Could you check a few things on this model? Use its own coordinates, in mm. Give positions to 0.01 mm unless a question says otherwise; leave off trailing zeros. Order: outer loops, then holes, each group sorted by start corner. A loop starts at its lowest first (then second) coordinate and runs counter-clockwise, first axis right, second up.
(1) If I drill on probe 1 along Y at (x, z) = (7.5, 3); probe 2 along Y at (x, z) = (58.55, 1.75); probe 3 along Y at (x, z) = (99.5, 1.5), over which ranges is the centre line in solid material (lowest first)?
(2) Imagine slicing it at B-B, the plane x = 207.01. Write out the boundary of the cut face in (y, z) (3 decimals), then the cut area to 3 significant figures.
(3) Imagine slicing it at A-A, the plane y = 44.9. State how many separate pieces and enclosed holes the cut face has, then the cut area to 3 significant figures.
(4) Imagine slicing it at D-D, the plane x = 149. Write out the boundary of the cut face in (y, z), then the cut area to 3 significant figures.
(5) Imagine slicing it at C-C, the plane y = 34. Write out the boundary of the cut face in (x, z), then the cut area to 3 significant figures.
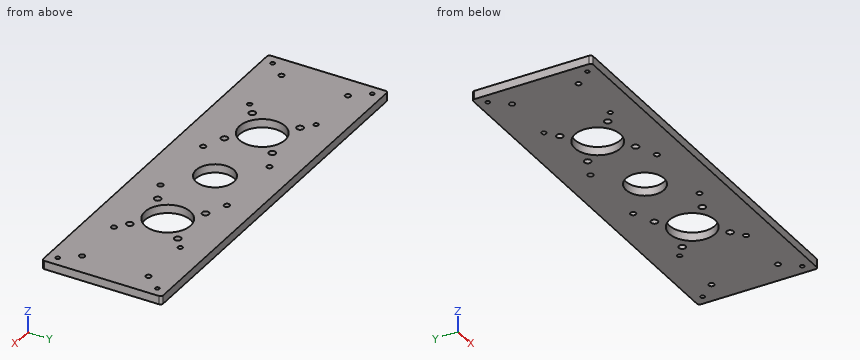
from build123d import *

# Parameters (mm, degrees)
SKETCH1_W           = 292.1
SKETCH1_H           = 89.8
SKETCH1_R           = 14.2875
SKETCH1_R_2         = 2.54
SKETCH1_R_3         = 17.145
BOSS_EXTRUDE1_DEPTH = 6.35
SKETCH2_R           = 2.05
CUT_EXTRUDE1_DEPTH  = 10
SKETCH3_R           = 1.55
SKETCH3_R_2         = 2.05
CUT_EXTRUDE2_DEPTH  = 10
FILLET1_R           = 2
SKETCH4_R           = 2.05
SKETCH4_R_2         = 1.778
CUT_EXTRUDE4_DEPTH  = 7.35


with BuildPart() as part:
    # Sketch1 → Boss-Extrude1 (new body)
    with BuildSketch(Plane.XY):
        with Locations((146.05, 44.9)):
            Rectangle(SKETCH1_W, SKETCH1_H)
        with Locations((146.05, 44.9)):
            Circle(SKETCH1_R, mode=Mode.SUBTRACT)
        with Locations((103.051585406, 62.859439014)):
            Circle(SKETCH1_R_2, mode=Mode.SUBTRACT)
        with Locations((103.049439014, 26.938414594)):
            Circle(SKETCH1_R_2, mode=Mode.SUBTRACT)
        with Locations((67.128414594, 26.940560986)):
            Circle(SKETCH1_R_2, mode=Mode.SUBTRACT)
        with Locations((67.130560986, 62.861585406)):
            Circle(SKETCH1_R_2, mode=Mode.SUBTRACT)
        with Locations((85.09, 44.9)):
            Circle(SKETCH1_R_3, mode=Mode.SUBTRACT)
        with Locations((189.050560986, 62.861585406)):
            Circle(SKETCH1_R_2, mode=Mode.SUBTRACT)
        with Locations((224.971585406, 62.859439014)):
            Circle(SKETCH1_R_2, mode=Mode.SUBTRACT)
        with Locations((224.969439014, 26.938414594)):
            Circle(SKETCH1_R_2, mode=Mode.SUBTRACT)
        with Locations((189.048414594, 26.940560986)):
            Circle(SKETCH1_R_2, mode=Mode.SUBTRACT)
        with Locations((207.01, 44.9)):
            Circle(SKETCH1_R_3, mode=Mode.SUBTRACT)
    extrude(amount=BOSS_EXTRUDE1_DEPTH)

    # Sketch2 → Cut-Extrude1 (cut)
    with BuildSketch(Plane.XY.offset(6.35)):
        with Locations((118.55, 20)):
            Circle(SKETCH2_R)
        with Locations((118.55, 69.8)):
            Circle(SKETCH2_R)
        with Locations((173.55, 20)):
            Circle(SKETCH2_R)
        with Locations((173.55, 69.8)):
            Circle(SKETCH2_R)
    extrude(amount=-CUT_EXTRUDE1_DEPTH, mode=Mode.SUBTRACT)

    # Sketch3 → Cut-Extrude2 (cut)
    with BuildSketch(Plane.XY.offset(6.35)):
        with Locations((284.6, 7.5)):
            Circle(SKETCH3_R)
        with Locations((7.5, 7.5)):
            Circle(SKETCH3_R)
        with Locations((7.5, 82.3)):
            Circle(SKETCH3_R)
        with Locations((284.6, 82.3)):
            Circle(SKETCH3_R)
        with Locations((274.6, 20)):
            Circle(SKETCH3_R_2)
        with Locations((17.5, 20)):
            Circle(SKETCH3_R_2)
        with Locations((17.5, 69.8)):
            Circle(SKETCH3_R_2)
        with Locations((274.6, 69.8)):
            Circle(SKETCH3_R_2)
    extrude(amount=-CUT_EXTRUDE2_DEPTH, mode=Mode.SUBTRACT)

    # Fillet1
    fillet1_edges = [part.edges().sort_by_distance(p)[0] for p in [
        (0, 89.8, 3.175),
        (292.1, 89.8, 3.175),
        (292.1, 0, 3.175),
        (0, 0, 3.175),
    ]]
    fillet(fillet1_edges, radius=FILLET1_R)

    # Sketch4 → Cut-Extrude4 (cut, through all)
    with BuildSketch(Plane.XY.offset(6.35)):
        with Locations((233.55, 20)):
            Circle(SKETCH4_R)
        with Locations((233.55, 69.8)):
            Circle(SKETCH4_R_2)
        with Locations((58.55, 69.8)):
            Circle(SKETCH4_R_2)
        with Locations((58.55, 20)):
            Circle(SKETCH4_R_2)
    extrude(amount=-CUT_EXTRUDE4_DEPTH, mode=Mode.SUBTRACT)


solid = part.part
Answer block:
1. probe 1: y = 0 to 5.95, 9.05 to 80.75, 83.85 to 89.8
1. probe 2: y = 0 to 18.22, 21.78 to 68.02, 71.58 to 89.8
1. probe 3: y = 0 to 35.61, 54.19 to 89.8
2. outline: (0, 0) - (27.755, 0) - (27.755, 6.35) - (0, 6.35) - close; (62.045, 0) - (89.8, 0) - (89.8, 6.35) - (62.045, 6.35) - close
2. area: 352 mm2
3. separate pieces: 4
3. enclosed holes: 0
3. area: 1,240 mm2
4. outline: (0, 0) - (30.92, 0) - (30.92, 6.35) - (0, 6.35) - close; (58.88, 0) - (89.8, 0) - (89.8, 6.35) - (58.88, 6.35) - close
4. area: 393 mm2
5. outline: (0, 0) - (71.86, 0) - (71.86, 6.35) - (0, 6.35) - close; (98.32, 0) - (136.81, 0) - (136.81, 6.35) - (98.32, 6.35) - close; (155.29, 0) - (193.78, 0) - (193.78, 6.35) - (155.29, 6.35) - close; (220.24, 0) - (292.1, 0) - (292.1, 6.35) - (220.24, 6.35) - close
5. area: 1,400 mm2
